The drawing under review shows one solid part. Ordinate dimensions are in mm from its lowest x, y, z. A direction names the side the tool comes from. Give positions to 0.01 mm unless a question says otherwise; leave off trailing zeros. Loops run counter-clockwise (first coordinate to the right, second up) from the corner with the lowest first, then second, coordinate; pieces in that order, holes last. Notation, with made-up numbers: (39.5, 62) -> (44.5, 62) arc R17 ccw to (44.5, 86) -> close; hole circle Ø8 at (15.25, -10.75). An arc over 180 degrees is marked (long way). Answer in a Markdown table with one row per item. Add a question column.
(1) For the marked faces 1 and 2, list the 3-axis set-ups (+Z, -Z, +X, -X, +Y, -Y) from which the entire face can be reached by the end or side of a thin tool; tool diameter is ignored.
(2) Consider section B-B on x = 1.75. Write out the cut boundary in (y, z), then the cut area to 3 significant figures.
(3) For pin 1 (1.5 mm diameter, centred on x = 2.5, y = 1, fed in from -Z); pin 2 (1.5 mm diameter, centred on y = 3.5, z = 4.5, fed in from +X); pin 3 (1 mm diameter, centred on x = 2.5, y = 1.5, fed in from -Z), all flat-tipped, find the tip position at first contact; note any pin that passes through.
(4) Consider section C-C on z = 4.5. Write out the cut boundary in (x, y).
(5) For line 1 (X direction, y = 3.05, z = 6.5); line 2 (Z direction, x = 2.05, y = 0.9); line 3 (X direction, y = 2.3, z = 1.25), list the stretches that pass through material, from the lowest coordinate up.
(6) Consider section A-A on y = 3.55. Write out the cut boundary in (x, z).
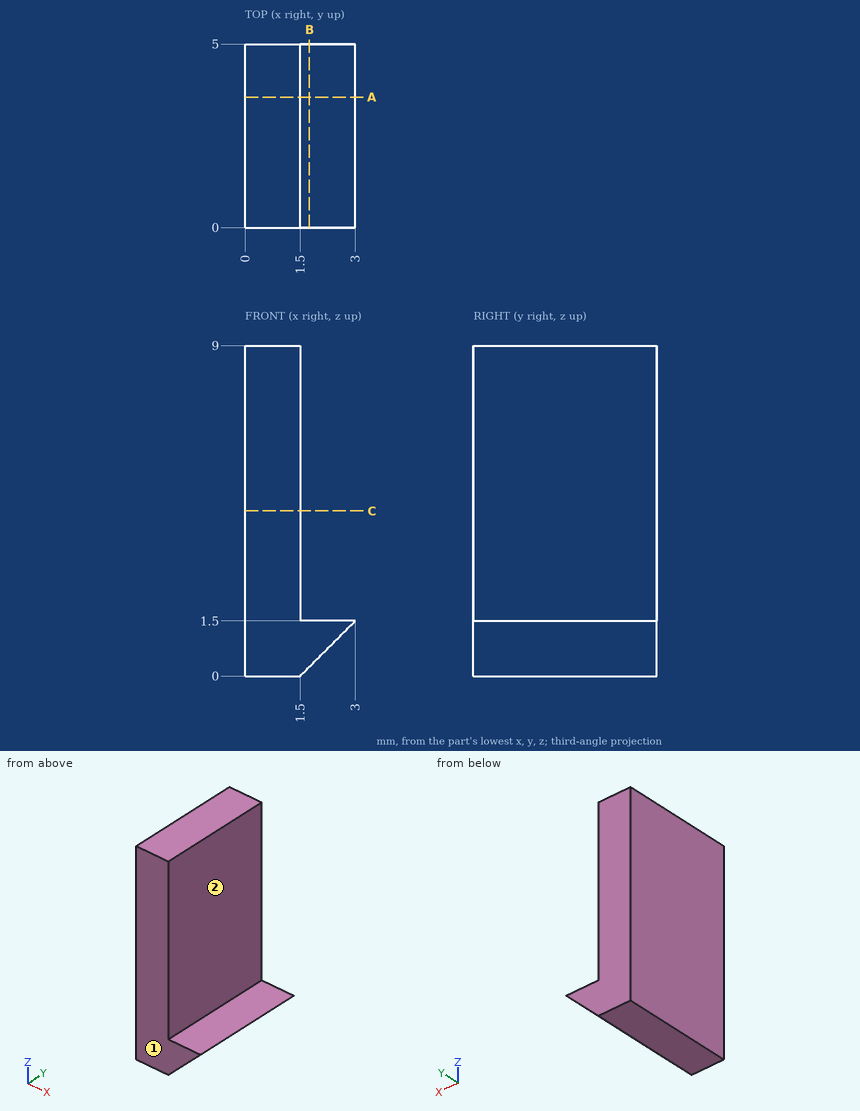
Values follow:
| question | item | result |
|---|---|---|
| 1 | face 1 | +Z, -Z, +X, -X, -Y |
| 1 | face 2 | +Z, +X, +Y, -Y |
| 2 | outline | (0, 0.25) -> (5, 0.25) -> (5, 1.5) -> (0, 1.5) -> close |
| 2 | area | 6.25 mm2 |
| 3 | pin 1 | z = 0.25 |
| 3 | pin 2 | x = 1.5 |
| 3 | pin 3 | z = 0.5 |
| 4 | outline | (0, 0) -> (1.5, 0) -> (1.5, 5) -> (0, 5) -> close |
| 5 | line 1 | 0 to 1.5 |
| 5 | line 2 | 0.55 to 1.5 |
| 5 | line 3 | 0 to 2.75 |
| 6 | outline | (0, 0) -> (1.5, 0) -> (3, 1.5) -> (1.5, 1.5) -> (1.5, 9) -> (0, 9) -> close |
